```python
from build123d import *

# Parameters (mm, degrees)
SKETCH1_R               = 1.5
BASE_EXTRUDE_DEPTH      = 3.5
DOME1_FACE_RADIUS       = 1.5
DOME1_HEIGHT            = 1.5
SKETCH2_R               = 2
BOSS_EXTRUDE1_DEPTH     = 1
SKETCH3_W               = 0.2
SKETCH3_H               = 0.5
BOSS_EXTRUDE2_DEPTH     = 5
CUT_EXTRUDE1_DEPTH      = 6
CUT_EXTRUDE1_DEPTH_BACK = 7


with BuildPart() as part:
    # Sketch1 → Base-Extrude (new body)
    with BuildSketch(Plane.XY):
        Circle(SKETCH1_R)
    extrude(amount=BASE_EXTRUDE_DEPTH)

    # Dome1: a dome of height H over a round flat face of radius A is a cap of a sphere of radius (A * A + H * H) / (2 * H)
    dome1_r = (DOME1_FACE_RADIUS * DOME1_FACE_RADIUS + DOME1_HEIGHT * DOME1_HEIGHT) / (2 * DOME1_HEIGHT)
    dome1_base = Plane((0, 0, 3.5), z_dir=(0, 0, 1))
    with Locations(dome1_base.offset(DOME1_HEIGHT - dome1_r)):
        dome1_ball = Sphere(dome1_r, mode=Mode.PRIVATE)
    add(split(dome1_ball, bisect_by=dome1_base, keep=Keep.TOP, mode=Mode.PRIVATE))

    # Sketch2 → Boss-Extrude1 (add)
    with BuildSketch(Plane(origin=(0, 0, 0), x_dir=(-1, 0, 0), z_dir=(0, 0, -1))):
        Circle(SKETCH2_R)
    extrude(amount=BOSS_EXTRUDE1_DEPTH)

    # Sketch3 → Boss-Extrude2 (add)
    with BuildSketch(Plane(origin=(0, 0, -1), x_dir=(-1, 0, 0), z_dir=(0, 0, -1))):
        with Locations((0, 1.25)):
            Rectangle(SKETCH3_W, SKETCH3_H)
        with Locations((0, -1.25)):
            Rectangle(SKETCH3_W, SKETCH3_H)
    extrude(amount=BOSS_EXTRUDE2_DEPTH)

    # Sketch5 → Cut-Extrude1 (cut, two sides)
    with BuildSketch(Plane(origin=(0, 0, -1), x_dir=(-1, 0, 0), z_dir=(0, 0, -1))) as cut_extrude1_sk:
        Polygon((-20.975129822, 1.5), (-1.322875656, 1.5), (1.322875656, 1.5), (20.975129822, 1.5), (20.975129822, 40.804508332), (-20.975129822, 40.804508332), align=None)
    extrude(amount=CUT_EXTRUDE1_DEPTH, mode=Mode.SUBTRACT)
    extrude(cut_extrude1_sk.sketch, amount=-CUT_EXTRUDE1_DEPTH_BACK, mode=Mode.SUBTRACT)


solid = part.part
```
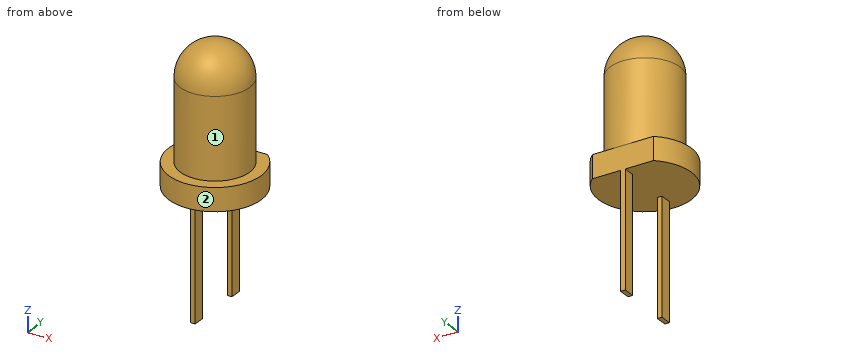
Input: part model. Units: mm. Frame: model coordinates. Face numbers are marked on the shaded views. A direction names the side the tool comes from. Give positions to 0.01 mm unless a question says otherwise; leave off trailing zeros. Order: outer loops, then holes, each group sorted by start corner. A loop starts at its lowest first (then second) coordinate and runs counter-clockwise, first axis right, second up.
1. Section C-C on x = -1. Return the cut outline in (y, z), and give its area (3 significant figures).
Derived:
outline: (-1.73, -1) - (1.5, -1) - (1.5, 0) - (1.12, 0) - (1.12, 3.5) arc R1.12 ccw to (-1.12, 3.5) - (-1.12, 0) - (-1.73, 0) - close
area: 13.0 mm2
2. Section B-B on y = 0. Return the cut outline in (x, z), and give its area (3 significant figures).
Derived:
outline: (-2, -1) - (2, -1) - (2, 0) - (1.5, 0) - (1.5, 3.5) arc R1.5 ccw to (-1.5, 3.5) - (-1.5, 0) - (-2, 0) - close
area: 18.0 mm2
3. Section A-A on z = -2.5. Return the cut outline in (x, y), and give its area (3 significant figures).
Derived:
outline: (-0.1, -1.5) - (0.1, -1.5) - (0.1, -1) - (-0.1, -1) - close; (-0.1, 1) - (0.1, 1) - (0.1, 1.5) - (-0.1, 1.5) - close
area: 0.200 mm2
4. Material intervals for L1, parallel to Z at x = 0.9, y = -1.5; L2, parallel to X at y = 1.35, z = 2.25; L3, parallel to X at y = 0.25, z = -0.25, sorted ascending.
Derived:
L1: z = -1 to 0
L2: x = -0.65 to 0.65
L3: x = -1.98 to 1.98
5. Reachability of the marked faces 1 and 2 from +Z, -Z, +X, -X, +Y, -Y: full face, straight path, thin tool, end or side. Return the list, or none.
Derived:
face 1: +Z
face 2: +Z, -Z
6. Section D-D on z = 0.5. Return the cut outline in (x, y), and give its area (3 significant figures).
Derived:
outline: circle Ø3 at (0, 0)
area: 7.07 mm2
7. Pin query (flat end, axial travel): pin 1 (0.6 mm diameter, centred on y = -1, z = -3.5, fed in from +X); pin 2 (1 mm diameter, centred on x = -0.5, y = 0.5, fed in from +Z); pin 3 (1.5 mm diameter, centred on x = 0.5, z = -2.5, fed in from +Y). Return the tip coordinate at first contact, or that it passes through.
Derived:
pin 1: stops at x = 0.1
pin 2: stops at z = 4.99
pin 3: stops at y = 1.5
